Here's how the part is built. I have some questions about the finished solid (model axes, mm). Face numbers are marked on the shaded views. A direction names the side the tool comes from. Coordinates: 2 decimals unless noted, no trailing zeros. Write each loop counter-clockwise with the first axis right and the second up, starting at its lowest first coordinate (ties: lowest second). Pieces come first, ordered by that corner, then holes. Notation, with made-up numbers: M 37,61 L 58,61 A6 cw 58,69 Z; hole C 71.5,78 d3. An arc over 180 degrees is marked long. Use one line per item in the form item = value. Start each with the question number.
1. I want a section at A-A, the plane y = 0. List the corners of the cut face in (x, z) for me (3 decimals).
2. Please list where these lines run through material, in increasing order: line 1 along Y through (x, z) = (3.5, 5.25); line 2 along Y through (x, z) = (0, 3.75) (3 decimals); line 3 along Y through (x, z) = (-2, 3.5). Write a range as [from, to].
3. Thinking about a two-plate mould opening in X: for the marked faces 1, 2 and 3, which applies, released by +X, released by -X, zero draft, split by the parting line, or undercut?
4. I want a section at C-C, the plane x = -5. List the corners of the cut face in (y, z) for me, plus the area to 3 significant figures.
5. I want a section at B-B, the plane x = 0. List the corners of the cut face in (y, z) for me (3 decimals).
6. On a 3-axis mill with a long thin cutter (end or side, diameter ignored), from which of +Z, -Z, +X, -X, +Y, -Y can I reach the whole of each face in a straight line? I mean the marked faces 4, 5 and 6. Say none if no direction works.
7. I'm going to push flat-ended pins straight in: pin 1 Ø1.8 at (x, z) = (3, 2.5) entering from -Y; pin 2 Ø5 at (x, y) = (-14.5, 3.5) entering from -Z. Where does each tip first touch, or does it pass through?
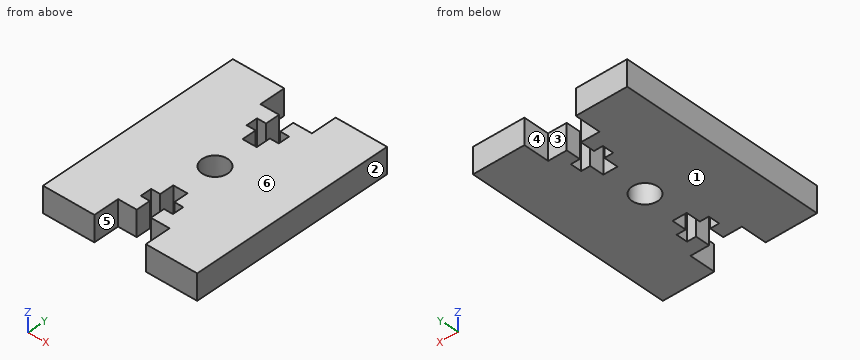
from build123d import *

# Parameters (mm, degrees)
BOSS_EXTRUDE1_DEPTH = 6.35
SKETCH3_R           = 3.175
CUT_EXTRUDE1_DEPTH  = 33.378773911


with BuildPart() as part:
    # Sketch2 → Boss-Extrude1 (new body)
    with BuildSketch(Plane.XY):
        Polygon((-19.05, 0), (-19.05, 25.4), (-6.35, 25.4), (-6.35, 19.05), (-1.7526, 19.05), (-1.7526, 15.5495625), (-3.96875, 15.5495625), (-3.96875, 12.7714375), (-1.7526, 12.7714375), (-1.7526, 9.271), (1.7526, 9.271), (1.7526, 12.7714375), (3.96875, 12.7714375), (3.96875, 15.5495625), (1.7526, 15.5495625), (1.7526, 19.05), (6.35, 19.05), (6.35, 25.4), (19.05, 25.4), (19.05, 0), align=None)
    boss_extrude1 = extrude(amount=BOSS_EXTRUDE1_DEPTH)

    # Mirror1: Boss-Extrude1 across plane
    add(boss_extrude1.mirror(Plane(origin=(-19.05, 0, 6.35), x_dir=(0, 0, 1), z_dir=(0, 1, 0))))

    # Sketch3 → Cut-Extrude1 (cut, through all)
    with BuildSketch(Plane.XY.offset(6.35)):
        Circle(SKETCH3_R)
    extrude(amount=-CUT_EXTRUDE1_DEPTH, mode=Mode.SUBTRACT)


solid = part.part
Answer list:
q1.outline = M -19.05,0 L -3.175,0 L -3.175,6.35 L -19.05,6.35 Z; M 3.175,0 L 19.05,0 L 19.05,6.35 L 3.175,6.35 Z
q2.line_1 = [-19.05, -15.55], [-12.77, 12.77], [15.55, 19.05]
q2.line_2 = [-9.271, -3.175], [3.175, 9.271]
q2.line_3 = [-19.05, -15.55], [-12.77, -2.47], [2.47, 12.77], [15.55, 19.05]
q3.face_1 = zero draft
q3.face_2 = released by +X
q3.face_3 = undercut
q4.outline = M -19.05,0 L 19.05,0 L 19.05,6.35 L -19.05,6.35 Z
q4.area = 242 mm²
q5.outline = M -9.271,0 L -3.175,0 L -3.175,6.35 L -9.271,6.35 Z; M 3.175,0 L 9.271,0 L 9.271,6.35 L 3.175,6.35 Z
q6.face_4 = +Z, -Z, +Y
q6.face_5 = +Z, -Z, -Y
q6.face_6 = +Z, +X, -X, +Y, -Y
q7.pin_1 = -19.05
q7.pin_2 = 0
